Verification items for the finished model (mm, model axes). Round coordinates to 2 decimals unless told otherwise and drop trailing zeros. Order: outer loops, then holes, each group sorted by start corner. A loop starts at its lowest first (then second) coordinate and runs counter-clockwise, first axis right, second up. Notation, with made-up numbers: (52, 84) -> (77, 84) arc R18 ccw to (77, 113) -> close; hole circle Ø10 at (72.25, 80). An arc over 180 degrees is marked (long way). Put each result on its own line as item: value.
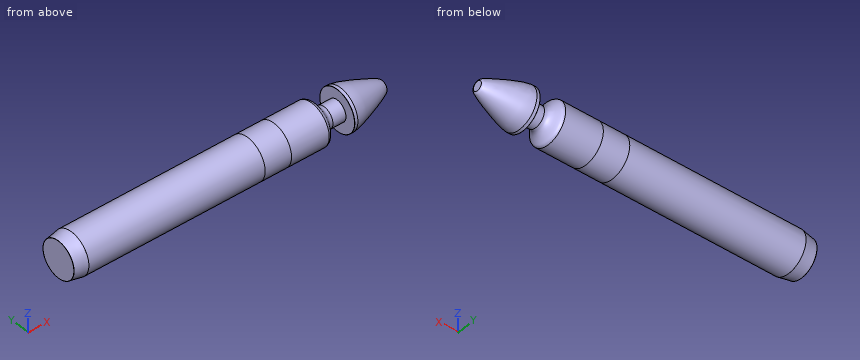
from build123d import *

# Parameters (mm, degrees)
BREAK_EDGES_R = 0.02


with BuildPart() as part:
    # body_sketch → body (revolve)
    with BuildSketch(Plane.XY):
        with BuildLine():
            Line((-16.73571407, 3.175), (-10.921788615, 3.175))
            add(Edge.make_bspline(
                [(-10.921788615, 3.175), (-10.165447426, 3.175), (-10.250040485, 1.5875), (-9, 1.5875)],
                knots=[0, 0, 0, 0, 1, 1, 1, 1], degree=3))
            Line((-9, 1.5875), (-7, 1.5875))
            Line((-7, 1.5875), (-7, 3.175))
            Line((-7, 3.175), (-6.5, 3.175))
            add(Edge.make_bspline(
                [(-6.5, 3.175), (-5.484084378, 3.175), (-0.421041724, 1.302274259), (-0.009654297, 0.817143972), (0, 0.774017781), (0, 0.724579725)],
                knots=[0, 0, 0, 0, 0.586137631, 0.686137631, 1, 1, 1, 1], degree=3))
            Line((0, 0.724579725), (0, 0))
            Line((0, 0), (-50, 0))
            Line((-50, 0), (-50, 2.822346039))
            Line((-50, 2.822346039), (-48, 3.175))
            Line((-48, 3.175), (-20.811079947, 3.175))
            add(Edge.make_bspline(
                [(-20.811079947, 3.175), (-19.383200887, 3.175), (-18.073641119, 3.175), (-16.73571407, 3.175)],
                knots=[0, 0, 0, 0, 1, 1, 1, 1], degree=3))
        make_face()
    revolve(axis=Axis((0, 0, 0), (-1, 0, 0)))

    # break_edges
    break_edges_edges = [part.edges().sort_by_distance(p)[0] for p in [
        (-7, -3.175, 0),
        (-50, -2.822346039, 0),
        (-48, -3.175, 0),
    ]]
    fillet(break_edges_edges, radius=BREAK_EDGES_R)


solid = part.part
Item 1: Gauge pin test, flat ends, axial feed: pin 1 Ø2 at (x, z) = (-38, -1.5) entering from -Y; pin 2 Ø3 at (y, z) = (1, 2) entering from +X. Record the tip position at first contact, or that the pin passes through.
Check sheet entries:
pin 1: stops at y = -3.14
pin 2: stops at x = 0
Item 2: Material ranges on L1, parallel to Z at x = -36.5, y = 1.5; L2, parallel to Z at x = -26.5, y = -1.75; L3, parallel to Y at x = -44, z = -1, recorded low to high. Write a range as [from, to].
Check sheet entries:
L1: z = [-2.8, 2.8]
L2: z = [-2.65, 2.65]
L3: y = [-3.01, 3.01]
Item 3: Section check A-A on x = -27. Record the boundary of the cut face in (y, z) (3 decimals), then the cut area to 3 significant figures.
Check sheet entries:
outline: circle Ø6.35 at (0, 0)
area: 31.7 mm^2
